Could you check a few things on this model? Use its own coordinates, in mm. Give positions to 0.01 mm unless a question says otherwise; leave off trailing zeros. Write each loop counter-clockwise with the first axis right and the second up, starting at its lowest first coordinate (ties: lowest second). Pieces come first, ordered by that corner, then holes. Notation, with made-up numbers: (-30.75, 76.25) - (-18.75, 76.25) arc R33 cw to (-18.75, 108.25) - close; hole circle Ø1 at (77.25, 23). An arc over 180 degrees is marked (long way). Answer as CSV lines item,"result". Start each with the question number.
Q1. Imagine slicing it at B-B on y = -1. List the corners of the cut face in (x, z) for me.
Q2. If I drill on line 1 along Y through (x, z) = (82, -10.5); line 2 along Y through (x, z) = (22, 14.5); line 3 along Y through (x, z) = (18, -17), over which ranges is the centre line in solid material (lowest first)?
Q3. Imagine slicing it at A-A on z = -19. List the corners of the cut face in (x, y) for me, and give its area (3 significant figures).
Q4. Will these pins go through, and if not, where does the flat tip stop? pin 1 Ø1.2 at (x, z) = (53, -8.5) entering from +Y; pin 2 Ø0.6 at (x, y) = (47.5, 22.5) entering from +Z.
Q5. Imagine slicing it at C-C on z = -3. List the corners of the cut face in (x, y) for me.
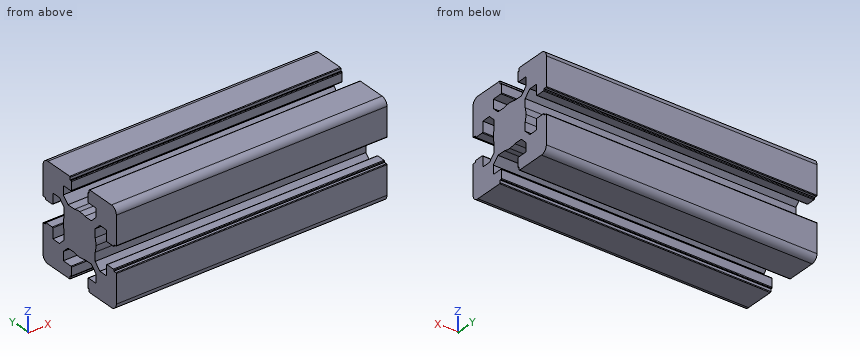
```python
from build123d import *

# Parameters (mm, degrees)
F1_DEPTH = 127


with BuildPart() as f1:
    # F0 (on Right) → F1 (new body)
    with BuildSketch(Plane.YZ):
        with BuildLine():
            Line((-20.088481, -9.788837), (-20.088481, -10.288837))
            Line((-20.088481, -10.288837), (-21.28859, -10.288837))
            ThreePointArc((-21.28859, -10.288837), (-21.500722, -10.376705), (-21.58859, -10.588837))
            Line((-21.58859, -10.588837), (-21.58859, -23.988949))
            ThreePointArc((-21.58859, -23.988949), (-20.70991, -26.11027), (-18.58859, -26.988949))
            Line((-18.58859, -26.988949), (-5.188544, -26.988949))
            ThreePointArc((-5.188544, -26.988949), (-4.976411, -26.901081), (-4.888544, -26.688949))
            Line((-4.888544, -26.688949), (-4.888544, -25.488841))
            Line((-4.888544, -25.488841), (-4.388544, -25.488841))
            ThreePointArc((-4.388544, -25.488841), (-4.176411, -25.400973), (-4.088544, -25.188841))
            Line((-4.088544, -25.188841), (-4.088544, -21.288841))
            ThreePointArc((-4.088544, -21.288841), (-4.176411, -21.076709), (-4.388544, -20.988841))
            Line((-4.388544, -20.988841), (-9.138663, -20.988841))
            Line((-9.138663, -20.988841), (-9.138663, -16.881665))
            Line((-9.138663, -16.881665), (-6.245729, -13.988731))
            Line((-6.245729, -13.988731), (-2.211433, -13.988731))
            ThreePointArc((-2.211433, -13.988731), (-0.669869, -14.363044), (0.91149, -14.48887))
            Line((0.91149, -14.48887), (0.91149, -4.48887))
            Line((0.91149, -4.48887), (-9.08851, -4.48887))
            ThreePointArc((-9.08851, -4.48887), (-8.962684, -6.070229), (-8.588371, -7.611793))
            Line((-8.588371, -7.611793), (-8.588371, -11.646022))
            Line((-8.588371, -11.646022), (-11.481305, -14.538956))
            Line((-11.481305, -14.538956), (-15.588481, -14.538956))
            Line((-15.588481, -14.538956), (-15.588481, -9.788837))
            ThreePointArc((-15.588481, -9.788837), (-15.676349, -9.576705), (-15.888481, -9.488837))
            Line((-15.888481, -9.488837), (-19.788481, -9.488837))
            ThreePointArc((-19.788481, -9.488837), (-20.000613, -9.576705), (-20.088481, -9.788837))
        make_face()
        with BuildLine():
            ThreePointArc((-8.588371, -1.365947), (-8.962684, -2.907511), (-9.08851, -4.48887))
            Line((-9.08851, -4.48887), (0.91149, -4.48887))
            Line((0.91149, -4.48887), (0.91149, 5.51113))
            ThreePointArc((0.91149, 5.51113), (-0.669869, 5.385303), (-2.211433, 5.010991))
            Line((-2.211433, 5.010991), (-6.245729, 5.010991))
            Line((-6.245729, 5.010991), (-9.138663, 7.903925))
            Line((-9.138663, 7.903925), (-9.138663, 12.011101))
            Line((-9.138663, 12.011101), (-4.388544, 12.011101))
            ThreePointArc((-4.388544, 12.011101), (-4.176411, 12.098969), (-4.088544, 12.311101))
            Line((-4.088544, 12.311101), (-4.088544, 16.211101))
            ThreePointArc((-4.088544, 16.211101), (-4.176411, 16.423233), (-4.388544, 16.511101))
            Line((-4.388544, 16.511101), (-4.888544, 16.511101))
            Line((-4.888544, 16.511101), (-4.888544, 17.711209))
            ThreePointArc((-4.888544, 17.711209), (-4.976411, 17.923341), (-5.188544, 18.011209))
            Line((-5.188544, 18.011209), (-18.58859, 18.011209))
            ThreePointArc((-18.58859, 18.011209), (-20.70991, 17.13253), (-21.58859, 15.011209))
            Line((-21.58859, 15.011209), (-21.58859, 1.611097))
            ThreePointArc((-21.58859, 1.611097), (-21.500722, 1.398965), (-21.28859, 1.311097))
            Line((-21.28859, 1.311097), (-20.088481, 1.311097))
            Line((-20.088481, 1.311097), (-20.088481, 0.811097))
            ThreePointArc((-20.088481, 0.811097), (-20.000613, 0.598965), (-19.788481, 0.511097))
            Line((-19.788481, 0.511097), (-15.888481, 0.511097))
            ThreePointArc((-15.888481, 0.511097), (-15.676349, 0.598965), (-15.588481, 0.811097))
            Line((-15.588481, 0.811097), (-15.588481, 5.561216))
            Line((-15.588481, 5.561216), (-11.481305, 5.561216))
            Line((-11.481305, 5.561216), (-8.588371, 2.668282))
            Line((-8.588371, 2.668282), (-8.588371, -1.365947))
        make_face()
        with BuildLine():
            Line((0.91149, 5.51113), (0.91149, -4.48887))
            Line((0.91149, -4.48887), (10.91149, -4.48887))
            ThreePointArc((10.91149, -4.48887), (10.785663, -2.907511), (10.41135, -1.365947))
            Line((10.41135, -1.365947), (10.41135, 2.668282))
            Line((10.41135, 2.668282), (13.304285, 5.561216))
            Line((13.304285, 5.561216), (14.016842, 5.561216))
            Line((14.016842, 5.561216), (17.41146, 5.561216))
            Line((17.41146, 5.561216), (17.41146, 0.811097))
            ThreePointArc((17.41146, 0.811097), (17.499328, 0.598965), (17.71146, 0.511097))
            Line((17.71146, 0.511097), (21.61146, 0.511097))
            ThreePointArc((21.61146, 0.511097), (21.823593, 0.598965), (21.91146, 0.811097))
            Line((21.91146, 0.811097), (21.91146, 1.311097))
            Line((21.91146, 1.311097), (23.111569, 1.311097))
            ThreePointArc((23.111569, 1.311097), (23.323701, 1.398965), (23.411569, 1.611097))
            Line((23.411569, 1.611097), (23.411569, 15.011209))
            ThreePointArc((23.411569, 15.011209), (22.532889, 17.13253), (20.411569, 18.011209))
            Line((20.411569, 18.011209), (7.011523, 18.011209))
            ThreePointArc((7.011523, 18.011209), (6.799391, 17.923341), (6.711523, 17.711209))
            Line((6.711523, 17.711209), (6.711523, 16.511101))
            Line((6.711523, 16.511101), (6.211523, 16.511101))
            ThreePointArc((6.211523, 16.511101), (5.999391, 16.423233), (5.911523, 16.211101))
            Line((5.911523, 16.211101), (5.911523, 12.311101))
            ThreePointArc((5.911523, 12.311101), (5.999391, 12.098969), (6.211523, 12.011101))
            Line((6.211523, 12.011101), (10.961642, 12.011101))
            Line((10.961642, 12.011101), (10.961642, 7.903925))
            Line((10.961642, 7.903925), (8.068708, 5.010991))
            Line((8.068708, 5.010991), (4.034413, 5.010991))
            ThreePointArc((4.034413, 5.010991), (2.492849, 5.385303), (0.91149, 5.51113))
        make_face()
        with BuildLine():
            Line((10.91149, -4.48887), (0.91149, -4.48887))
            Line((0.91149, -4.48887), (0.91149, -14.48887))
            ThreePointArc((0.91149, -14.48887), (2.492849, -14.363044), (4.034413, -13.988731))
            Line((4.034413, -13.988731), (8.068708, -13.988731))
            Line((8.068708, -13.988731), (10.961642, -16.881665))
            Line((10.961642, -16.881665), (10.961642, -20.988841))
            Line((10.961642, -20.988841), (6.211523, -20.988841))
            ThreePointArc((6.211523, -20.988841), (5.999391, -21.076709), (5.911523, -21.288841))
            Line((5.911523, -21.288841), (5.911523, -25.188841))
            ThreePointArc((5.911523, -25.188841), (5.999391, -25.400973), (6.211523, -25.488841))
            Line((6.211523, -25.488841), (6.711523, -25.488841))
            Line((6.711523, -25.488841), (6.711523, -26.688949))
            ThreePointArc((6.711523, -26.688949), (6.799391, -26.901081), (7.011523, -26.988949))
            Line((7.011523, -26.988949), (20.411569, -26.988949))
            ThreePointArc((20.411569, -26.988949), (22.532889, -26.11027), (23.411569, -23.988949))
            Line((23.411569, -23.988949), (23.411569, -10.588837))
            ThreePointArc((23.411569, -10.588837), (23.323701, -10.376705), (23.111569, -10.288837))
            Line((23.111569, -10.288837), (21.91146, -10.288837))
            Line((21.91146, -10.288837), (21.91146, -9.788837))
            ThreePointArc((21.91146, -9.788837), (21.823593, -9.576705), (21.61146, -9.488837))
            Line((21.61146, -9.488837), (17.71146, -9.488837))
            ThreePointArc((17.71146, -9.488837), (17.499328, -9.576705), (17.41146, -9.788837))
            Line((17.41146, -9.788837), (17.41146, -14.538956))
            Line((17.41146, -14.538956), (13.304285, -14.538956))
            Line((13.304285, -14.538956), (10.41135, -11.646022))
            Line((10.41135, -11.646022), (10.41135, -7.611793))
            ThreePointArc((10.41135, -7.611793), (10.785663, -6.070229), (10.91149, -4.48887))
        make_face()
    extrude(amount=F1_DEPTH)


solid = f1.part
```
Conclusion:
1,outline,"(0, -14.3) - (127, -14.3) - (127, 5.33) - (0, 5.33) - close"
2,line 1,"-21.58 to -15.59, -8.59 to 10.41, 17.41 to 23.4"
2,line 2,"-21.59 to -4.09, 5.91 to 23.41"
2,line 3,"-21.59 to -9.14, 10.96 to 23.41"
3,outline,"(0, -21.59) - (127, -21.59) - (127, -9.14) - (0, -9.14) - close; (0, 10.96) - (127, 10.96) - (127, 23.41) - (0, 23.41) - close"
3,area,"3,160 mm^2"
4,pin 1,"y = 10.41"
4,pin 2,"z = 17.42"
5,outline,"(0, -8.98) - (127, -8.98) - (127, 10.8) - (0, 10.8) - close"
